Check sheet for the modelled part. Datum: model origin and axes. Units: mm. Coordinates: 2 decimals unless noted, no trailing zeros. Order: outer loops, then holes, each group sorted by start corner. A loop starts at its lowest first (then second) coordinate and runs counter-clockwise, first axis right, second up.
from build123d import *

# Parameters (mm, degrees)
BALAYAGE1_PROFILE_R = 5
ESQUISSE2_R         = 15
ESQUISSE2_R_2       = 10
BOSS_EXTRU_1_DEPTH  = 5


with BuildPart() as part:
    # Balayage1: sweep along a path in Esquisse1
    with BuildLine(Plane.XY) as balayage1_path:
        Line((-400, 0), (400, 0))
    # Balayage1 profile (on start of the path) → Balayage1 (sweep)
    with BuildSketch(Plane(origin=(-400, 0, 0), x_dir=(0, 0, 1), z_dir=(1, 0, 0))):
        Circle(BALAYAGE1_PROFILE_R)
    sweep(path=balayage1_path.line)

    # Esquisse2 → Boss.-Extru.1 (add)
    with BuildSketch(Plane(origin=(0, 0, 0), x_dir=(1, 0, 0), z_dir=(0, 1, 0))):
        with Locations((0, -15)):
            Circle(ESQUISSE2_R)
        with Locations(Location((0, -15, 0), (0, 0, 90))):
            Circle(ESQUISSE2_R_2, mode=Mode.SUBTRACT)
    extrude(amount=BOSS_EXTRU_1_DEPTH)


solid = part.part
(1) Cross-section at A-A (y = 2). Enter the section's corners in (x, z).
Filled in:
outline: (-400, -4.58) - (400, -4.58) - (400, 4.58) - (10.79, 4.58) arc R15 ccw (long way) to (-10.79, 4.58) - (-400, 4.58) - close; hole circle Ø20 at (0, 15)
(2) Cross-section at B-B (x = 91.5). Enter the section's corners in (y, z).
Filled in:
outline: circle Ø10 at (0, 0)
(3) Thickness scan on probe 1 along X at (y, z) = (1.45, 15); probe 2 along Z at (x, y) = (103, 1); probe 3 along Z at (x, y) = (330, -0.5). Record the ranges inside material, lowest first.
Filled in:
probe 1: x = -15 to -10, 10 to 15
probe 2: z = -4.9 to 4.9
probe 3: z = -4.97 to 4.97
(4) Release check for a two-part mould opening along X. For faces 1 (the cylindrical face through (-3, 2.46, 5.46)), 2 (the flat face through (3, 5, 25)) record: +X half, -X half, draft (parallel to the pull), parting line (faces both ways), or undercut.
Filled in:
face 1: undercut
face 2: draft
(5) Go/stop test with flat-tipped pins: P1, Ø12.5, axis at x = -3.5, z = 23.5, coming from the -Y side; P2, Ø4, axis at x = -61, y = 2, coming from the +Z side; P3, Ø4, axis at x = 311.5, z = 8.5, coming from the +Y side; P4, Ø1, axis at x = -65, y = -1.5, coming from the -Z side. Record where each tip stops, or that it passes through.
Filled in:
P1: stops at y = 0
P2: stops at z = 5
P3: passes through
P4: stops at z = -4.9
